Can you work these out from the drawing? Everything is in mm from the part's minimum corner. Give positions to 0.01 mm unless a question says otherwise; leave off trailing zeros. Loops run counter-clockwise (first coordinate to the right, second up) from the corner with the lowest first, then second, coordinate; pieces in that order, holes last. Notation, with made-up numbers: (43.25, 48.5) -> (50.25, 48.5) arc R20 ccw to (50.25, 64.5) -> close; hole circle Ø8 at (-31.75, -11). An arc over 180 degrees is marked (long way). Return JSON: item names as keys, results as strings. Group by question number.
Q1. Will these pins go through, and if not, where does the flat tip stop? pin 1 (1 mm diameter, centred on y = 39, z = 1, fed in from -X); pin 2 (4 mm diameter, centred on x = 99.6, y = 51.8, fed in from +Z).
Q2. I need wall thicknesses on line 1 along Y through (x, z) = (55, 1.2) (1 decimal); line 2 along X through (y, z) = (49, 1.35) (1 decimal); line 3 along Y through (x, z) = (60.5, 0.45) (1 decimal). Which ranges of each line are inside material? Lowest first, please. Write a range as [from, to].
Q3. Suppose I cut it at A-A, the plane z = 0.95. Count the separate pieces of the cut face and the enclosed holes in it, and give its area (3 significant figures).
Q4. Suppose I cut it at B-B, the plane y = 4. Please give me the cut outline in (x, z).
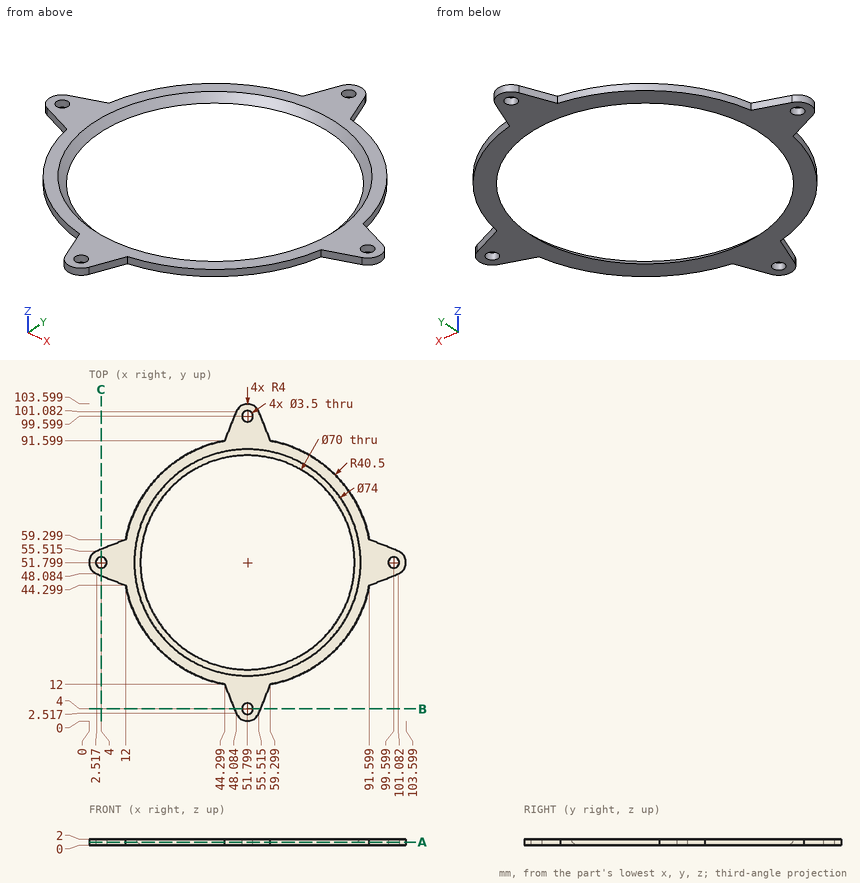
Ans:
{
 "1": {"pin 1": "stops at x = 13.21", "pin 2": "stops at z = 2"},
 "2": {"line 1": "y = [1.6, 15.7], [87.9, 102]", "line 2": "x = [1.1, 15.6], [88, 102.5]", "line 3": "y = [12.2, 17.4], [86.2, 91.4]"},
 "3": {"separate pieces": "1", "enclosed holes": "5", "area": "1,510 mm^2"},
 "4": {"outline": "(47.49, 0) -> (50.05, 0) -> (50.05, 2) -> (47.49, 2) -> close; (53.55, 0) -> (56.11, 0) -> (56.11, 2) -> (53.55, 2) -> close"}
}
